```python
from build123d import *

# Parameters (mm, degrees)
F0_W          = 31.7814054862
F0_H          = 6.2
F0_W_2        = 29.7814054862
F0_H_2        = 4.2
F1_DEPTH      = 5
F1_DEPTH_BACK = 5
F0_W_3        = 27.7814054862
F0_H_3        = 2.2
F2_DEPTH      = 10


with BuildPart() as f1:
    # F0 (on Front) → F1 (new body, two sides)
    with BuildSketch(Plane.XZ) as f1_sk:
        with Locations((-0.1092972569, 0)):
            Rectangle(F0_W, F0_H)
        with Locations((-0.1092972569, 0)):
            Rectangle(F0_W_2, F0_H_2, mode=Mode.SUBTRACT)
    extrude(amount=-F1_DEPTH)
    extrude(f1_sk.sketch, amount=F1_DEPTH_BACK)

    # F0 (on Front) → F2 (join)
    with BuildSketch(Plane.XZ):
        with Locations((-0.1092972569, 0)):
            Rectangle(F0_W_2, F0_H_2)
        with Locations((-0.1092972569, 0)):
            Rectangle(F0_W_3, F0_H_3, mode=Mode.SUBTRACT)
    extrude(amount=F2_DEPTH)


solid = f1.part
```
Can you work these out from the model? Positions are in its coordinate system, mm. A direction names the side the tool comes from. Give positions to 0.01 mm unless a question says otherwise; leave off trailing zeros. Loops run counter-clockwise (first coordinate to the right, second up) from the corner with the lowest first, then second, coordinate; pieces in that order, holes last. Notation, with made-up numbers: M 33.25,30.5 L 73.25,30.5 A21 cw 73.25,39.5 Z; hole C 44,81 d5. An arc over 180 degrees is marked long. One line per item, written item: value.
(1) We'd pull the mould along X, two halves only. Please class faces 4 (the face through (0, -7, 2.1)), 5 (the face through (-15, -7, 0)), 6 (the face through (-15, 3, 0)): released by +X, released by -X, zero draft, split by the parting line, or undercut.
Returned:
face 4: zero draft
face 5: released by -X
face 6: undercut
(2) Suppose I cut it at D-D on y = 1.25. List the corners of the cut face in (x, z) for me.
Returned:
outline: M -16,-3.1 L 15.78,-3.1 L 15.78,3.1 L -16,3.1 Z; hole M -15,-2.1 L 14.78,-2.1 L 14.78,2.1 L -15,2.1 Z
(3) Suppose I cut it at A-A on z = -0.75. List the corners of the cut face in (x, y) for me.
Returned:
outline: M -16,-5 L -15,-5 L -15,-10 L -14,-10 L -14,0 L -15,0 L -15,5 L -16,5 Z; M 13.78,-10 L 14.78,-10 L 14.78,-5 L 15.78,-5 L 15.78,5 L 14.78,5 L 14.78,0 L 13.78,0 Z
(4) Will these pins go through, and if not, where does the flat tip stop? pin 1 (4 mm diameter, centred on x = 3, y = -8.5, fed in from +Z); pin 2 (1.8 mm diameter, centred on y = -5.5, z = 0, fed in from +X); pin 3 (2 mm diameter, centred on x = -7.5, z = -1, fed in from +Y); pin 4 (1.5 mm diameter, centred on x = -0.5, y = -8, fed in from -Z).
Returned:
pin 1: z = 2.1
pin 2: x = 15.78
pin 3: y = 0
pin 4: z = -2.1
(5) Suppose I cut it at C-C on y = -2.5. List the corners of the cut face in (x, z) for me.
Returned:
outline: M -16,-3.1 L 15.78,-3.1 L 15.78,3.1 L -16,3.1 Z; hole M -14,-1.1 L 13.78,-1.1 L 13.78,1.1 L -14,1.1 Z
(6) I need wall thicknesses on line 1 (X direction, y = 2.5, z = -1); line 2 (Z direction, x = 4.5, y = 3.5); line 3 (X direction, y = -8.5, z = -1). Which ranges of each line are inside material? Lowest first, please.
Returned:
line 1: -16 to -15, 14.78 to 15.78
line 2: -3.1 to -2.1, 2.1 to 3.1
line 3: -15 to -14, 13.78 to 14.78
(7) Which directions (+Z, -Z, +X, -X, +Y, -Y) give clear straight access to the entire face, cutting with the end or side of a thin tool? Please do faces 1 (the face through (-0.3, 0, 1.4)), 2 (the face through (0, -5, 1.1)), 3 (the face through (14.781, -7, 0)).
Returned:
face 1: +Y
face 2: +Y, -Y
face 3: +Z, -Z, +X, -Y
(8) Suppose I cut it at B-B on x = -13.5. List the corners of the cut face in (y, z) for me.
Returned:
outline: M -10,-2.1 L -5,-2.1 L -5,-3.1 L 5,-3.1 L 5,-2.1 L 0,-2.1 L 0,-1.1 L -10,-1.1 Z; M -10,1.1 L 0,1.1 L 0,2.1 L 5,2.1 L 5,3.1 L -5,3.1 L -5,2.1 L -10,2.1 Z
